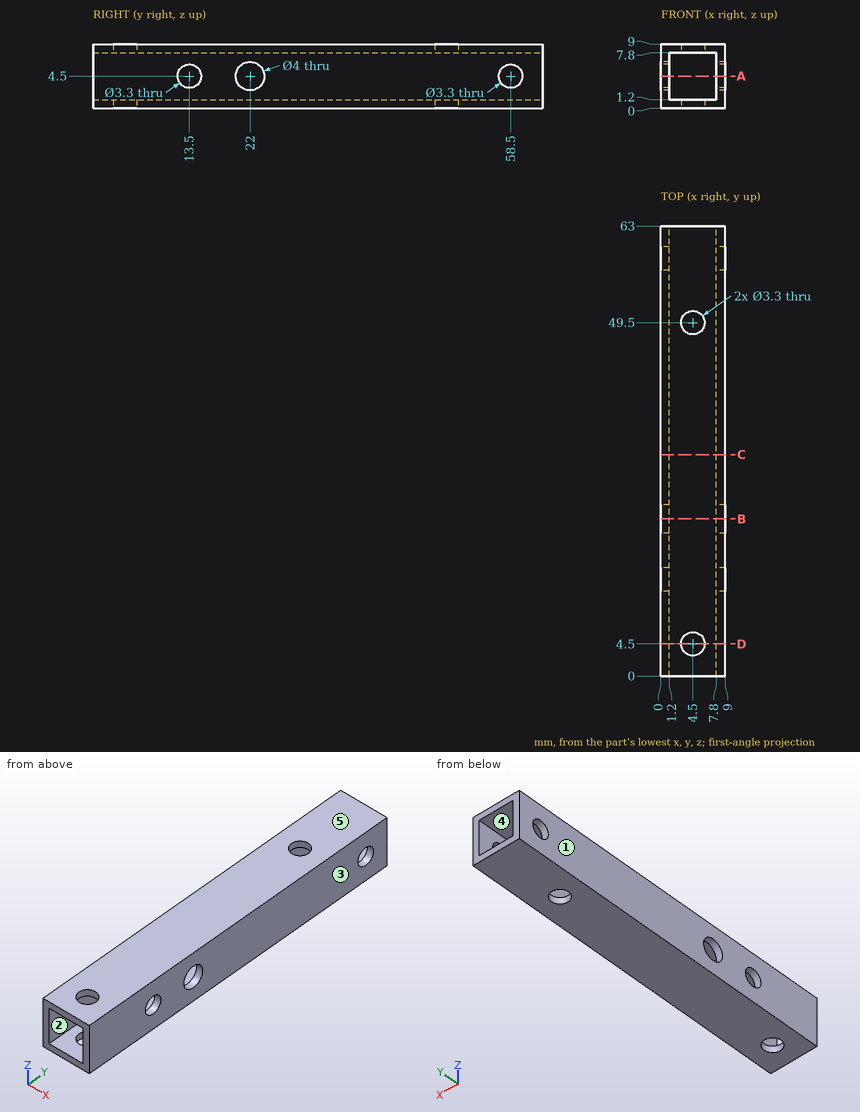
Could you check a few things on this drawing? It's one solid part, dimensions in mm from its lowest x, y, z. A direction names the side the tool comes from. Round coordinates to 2 decimals unless told otherwise and drop trailing zeros. Write each loop counter-clockwise with the first axis right and the second up, starting at its lowest first coordinate (ties: lowest second). Pieces come first, ordered by that corner, then holes. Notation, with made-up numbers: (37.25, -9) -> (55.25, -9) arc R27 cw to (55.25, 21) -> close; hole circle Ø8 at (34, -27). An arc over 180 degrees is marked (long way). One line per question, with ' | ' between items. Start each with the question number.
1) I need wall thicknesses on line 1 (Y direction, x = 0.3, z = 4.5); line 2 (X direction, y = 40, z = 4.75). Which ranges of each line are inside material? Lowest first, please. Write a range as [from, to].
2) Suppose I cut it at B-B on y = 22. Write out the boundary of the cut face in (x, z), then the cut area to 3 significant figures.
3) On a 3-axis mill with a long thin cutter (end or side, diameter ignored), from which of +Z, -Z, +X, -X, +Y, -Y can I reach the whole of each face in a straight line? I mean the marked faces 4 and 5. Say none if no direction works.
4) Suppose I cut it at C-C on y = 31. Write out the boundary of the cut face in (x, z), then the cut area to 3 significant figures.
5) If we mould it in two halves opening along X, with no side actions, what happens to the marked faces 1, 2 and 3? For each: released by +X, released by -X, zero draft, split by the parting line, or undercut.
6) Suppose I cut it at A-A on z = 4.5. Count the separate pieces of the cut face and the enclosed holes in it, then the cut area to 3 significant figures.
7) Suppose I cut it at D-D on y = 4.5. Write out the boundary of the cut face in (x, z).
Return value:
1) line 1: y = [0, 11.85], [15.15, 20], [24, 56.85], [60.15, 63] | line 2: x = [0, 1.2], [7.8, 9]
2) outline: (0, 0) -> (9, 0) -> (9, 2.5) -> (7.8, 2.5) -> (7.8, 1.2) -> (1.2, 1.2) -> (1.2, 2.5) -> (0, 2.5) -> close; (0, 6.5) -> (1.2, 6.5) -> (1.2, 7.8) -> (7.8, 7.8) -> (7.8, 6.5) -> (9, 6.5) -> (9, 9) -> (0, 9) -> close | area: 27.8 mm2
3) face 4: +Y, -Y | face 5: +Z, +X, -X, +Y, -Y
4) outline: (0, 0) -> (9, 0) -> (9, 9) -> (0, 9) -> close; hole (1.2, 1.2) -> (7.8, 1.2) -> (7.8, 7.8) -> (1.2, 7.8) -> close | area: 37.4 mm2
5) face 1: released by -X | face 2: undercut | face 3: released by +X
6) separate pieces: 8 | enclosed holes: 0 | area: 126 mm2
7) outline: (0, 0) -> (2.85, 0) -> (2.85, 1.2) -> (1.2, 1.2) -> (1.2, 7.8) -> (2.85, 7.8) -> (2.85, 9) -> (0, 9) -> close; (6.15, 0) -> (9, 0) -> (9, 9) -> (6.15, 9) -> (6.15, 7.8) -> (7.8, 7.8) -> (7.8, 1.2) -> (6.15, 1.2) -> close
